Print and shaded views of the part. All mm, measured from the part's lowest x, y and z. Round coordinates to 2 decimals unless told otherwise and drop trailing zeros. Write each loop counter-clockwise with the first axis right and the second up, starting at its lowest first coordinate (ties: lowest second). Pieces come first, ordered by that corner, then holes. Notation, with made-up numbers: (-19, -35) -> (18, -35) arc R14 cw to (18, -9) -> close; hole circle Ø8 at (13.25, -23). An arc over 180 degrees is marked (long way). Return JSON: item names as keys, results as strings. Group by question number.
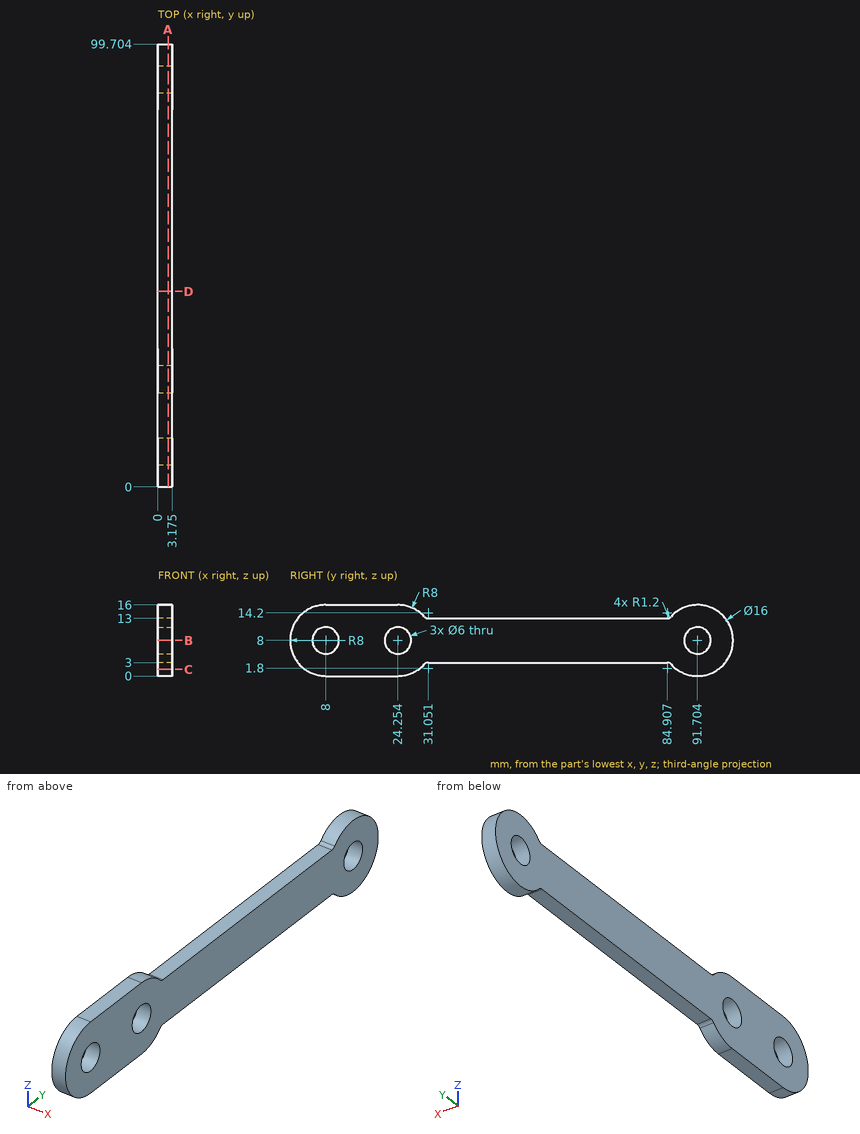
Item 1: Cut at A-A (x = 2.3). Write the cut outline in (y, z), then the cut area to 3 significant figures.
Item 2: Flat gauge pins, fed straight in: P1, Ø1.6, axis at x = 2, y = 47, coming from the -Z side; P2, Ø1.5, axis at x = 2, z = 11.5, coming from the -Y side; P3, Ø1, axis at x = 2, z = 12, coming from the -Y side. Where does each tip first touch, or does it go through?
Item 3: Wall check: L1, parallel to Z at x = 2.05, y = 8; L2, parallel to Y at x = 0.7, z = 7.5; L3, parallel to Z at x = 0.5, y = 53.5. Give the ranges that are in metal, low to high.
Item 4: Cut at B-B (z = 8). Write the cut outline in (x, y) (3 decimals), then the cut area to 3 significant figures.
Item 5: Cut at C-C (z = 1.5). Write the cut outline in (x, y) (3 decimals).
Item 6: Cut at D-D (y = 44). Write the cut outline in (x, z) (3 decimals).
Checks:
{
 "1": {"outline": "(8, 0) -> (24.25, 0) arc R8 ccw to (30.16, 2.61) arc R1.2 cw to (31.05, 3) -> (84.91, 3) arc R1.2 cw to (85.79, 2.61) arc R8 ccw (long way) to (85.79, 13.39) arc R1.2 cw to (84.91, 13) -> (31.05, 13) arc R1.2 cw to (30.16, 13.39) arc R8 ccw to (24.25, 16) -> (8, 16) arc R8 ccw to start; hole circle Ø6 at (8, 8); hole circle Ø6 at (24.25, 8); hole circle Ø6 at (91.7, 8)", "area": "1,100 mm2"},
 "2": {"P1": "stops at z = 3", "P2": "stops at y = 0.49", "P3": "stops at y = 0.81"},
 "3": {"L1": "z = 0 to 5, 11 to 16", "L2": "y = 0.02 to 5.04, 10.96 to 21.3, 27.21 to 88.75, 94.66 to 99.69", "L3": "z = 3 to 13"},
 "4": {"outline": "(0, 0) -> (3.175, 0) -> (3.175, 5) -> (0, 5) -> close; (0, 11) -> (3.175, 11) -> (3.175, 21.254) -> (0, 21.254) -> close; (0, 27.254) -> (3.175, 27.254) -> (3.175, 88.704) -> (0, 88.704) -> close; (0, 94.704) -> (3.175, 94.704) -> (3.175, 99.704) -> (0, 99.704) -> close", "area": "259 mm2"},
 "5": {"outline": "(0, 3.336) -> (3.175, 3.336) -> (3.175, 28.918) -> (0, 28.918) -> close; (0, 87.04) -> (3.175, 87.04) -> (3.175, 96.368) -> (0, 96.368) -> close"},
 "6": {"outline": "(0, 3) -> (3.175, 3) -> (3.175, 13) -> (0, 13) -> close"}
}
